Input: part model. Units: mm. Frame: model coordinates. Face numbers are marked on the shaded views. Coordinates: 2 decimals unless noted, no trailing zeros. Loops run counter-clockwise (first coordinate to the right, second up) from the corner with the lowest first, then second, coordinate; pieces in that order, holes last. Notation, with made-up numbers: (53, -21) -> (103, -21) arc R21 ccw to (103, 7) -> close; hole circle Ø4 at (-30, 47). An arc over 180 degrees is marked (long way). Put each result on its own line as item: value. Start each with the question number.
1) Material intervals for L1, parallel to Z at x = 10.25, y = -7.75; L2, parallel to Y at x = 9, z = -19.5; L3, parallel to X at y = 4.75, z = 15, sorted ascending.
2) Cut plane C-C (z = 2.5). Return the cut outline in (x, y), plus the area to 3 significant figures.
3) Pull-direction query (X, two-part tool) for the marked faces 1, 2, 3 and 4; classes: pulls with the +X half, pulls with the -X half, needs draft (parallel to the pull), parting line crosses it, or undercut.
4) Contact query for flat-ended pins moving along their axis: P1, Ø0.5, axis at x = 10.5, y = -2.5, coming from the +Z side; P2, Ø1, axis at x = 4.5, z = -5, coming from the -Y side; P3, Ø2, axis at y = 5, z = 14, coming from the +X side; P4, Ø2.5, axis at x = 11.5, y = -9.5, coming from the +Z side. Output: stop coordinate, or through.
5) Cut plane A-A (z = 15.5). Return the cut outline in (x, y), plus the area to 3 significant figures.
6) Cut plane D-D (x = 6). Return the cut outline in (y, z), plus the area to 4 significant figures.
7) Cut plane B-B (y = 7.25). Return the cut outline in (x, z), plus the area to 3 significant figures.
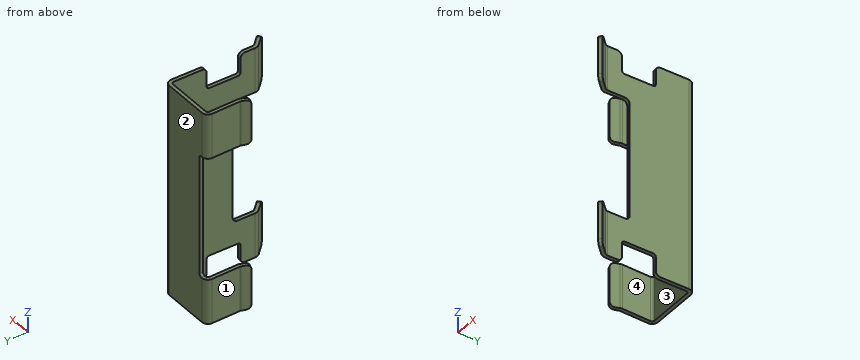
from build123d import *

# Parameters (mm, degrees)
BASE_FLANGE1_DEPTH = 22.5
CUT_EXTRUDE1_START = -9.35
CUT_EXTRUDE1_DEPTH = 9.35
CUT_EXTRUDE2_DEPTH = 28.952537171
FILLET_R1_R        = 1


# Read off the part's stored shape, not the designer's step: Cut-Extrude1
# Sheet-metal steps are written as plain solids
with BuildPart() as part:
    # Sketch1 → Base-Flange1 (new, symmetric)
    with BuildSketch(Plane.XY):
        with BuildLine():
            Line((-0.718242301, 0), (-0.090461069, 1.72481476))
            ThreePointArc((-0.090461069, 1.72481476), (-0.02278837, 1.977372708), (0, 2.237844975))
            Line((0, 2.237844975), (0, 8.1))
            ThreePointArc((0, 8.1), (0.146446609, 8.453553391), (0.5, 8.6))
            Line((0.5, 8.6), (9.985419886, 8.6))
            ThreePointArc((9.985419886, 8.6), (10.344017022, 8.448436644), (10.485213415, 8.085632378))
            Line((10.485213415, 8.085632378), (10.000619414, -8.771503263))
            ThreePointArc((10.000619414, -8.771503263), (10.098258212, -9.348572383), (10.409299492, -9.84434998))
            Line((10.409299492, -9.84434998), (12.522800458, -12.082961625))
            Line((12.522800458, -12.082961625), (13.068150712, -11.568089698))
            Line((13.068150712, -11.568089698), (10.954649746, -9.329478054))
            ThreePointArc((10.954649746, -9.329478054), (10.799129106, -9.081589256), (10.750309707, -8.793054696))
            Line((10.750309707, -8.793054696), (11.234903709, 8.064080946))
            ThreePointArc((11.234903709, 8.064080946), (10.881912725, 8.971091609), (9.985419886, 9.35))
            Line((9.985419886, 9.35), (0.5, 9.35))
            ThreePointArc((0.5, 9.35), (-0.383883476, 8.983883476), (-0.75, 8.1))
            Line((-0.75, 8.1), (-0.75, 2.237844975))
            ThreePointArc((-0.75, 2.237844975), (-0.761394185, 2.107608841), (-0.795230534, 1.981329867))
            Line((-0.795230534, 1.981329867), (-1.423011767, 0.256515107))
            Line((-1.423011767, 0.256515107), (-0.718242301, 0))
        make_face()
    extrude(amount=BASE_FLANGE1_DEPTH, both=True)

    # Cut-Extrude1 outline → Cut-Extrude1 (cut)
    with BuildSketch(Plane(origin=(0, 9.35, 0), x_dir=(-1, 0, 0), z_dir=(0, 1, 0)).offset(CUT_EXTRUDE1_START)):
        with BuildLine():
            ThreePointArc((-0.75, 13), (-1.103553391, 12.853553391), (-1.25, 12.5))
            Line((-1.25, 12.5), (-1.25, -12.5))
            ThreePointArc((-1.25, -12.5), (-1.103553391, -12.853553391), (-0.75, -13))
            Line((-0.75, -13), (3, -13))
            Line((3, -13), (3, 13))
            Line((3, 13), (-0.75, 13))
        make_face()
    extrude(amount=CUT_EXTRUDE1_DEPTH, mode=Mode.SUBTRACT)

    # Sketch5 → Cut-Extrude2 (cut, through all)
    with BuildSketch(Plane(origin=(10.244308957, -0.294494318, 0), x_dir=(0, 0, -1), z_dir=(0.999587057638364, -0.02873524320200468, 0))):
        with BuildLine():
            Line((-22.5, 1.533588636), (-18.5, 1.533588636))
            ThreePointArc((-18.5, 1.533588636), (-18.146446609, 1.387142026), (-18, 1.033588636))
            Line((-18, 1.033588636), (-18, -4.966411364))
            ThreePointArc((-18, -4.966411364), (-18.146446609, -5.319964755), (-18.5, -5.466411364))
            Line((-18.5, -5.466411364), (-22.5, -5.466411364))
            Line((-22.5, -5.466411364), (-22.5, 1.533588636))
        make_face()
        with BuildLine():
            Line((18, 1.033588636), (18, -4.966411364))
            ThreePointArc((18, -4.966411364), (18.146446609, -5.319964755), (18.5, -5.466411364))
            Line((18.5, -5.466411364), (22.5, -5.466411364))
            Line((22.5, -5.466411364), (22.5, 1.533588636))
            Line((22.5, 1.533588636), (18.5, 1.533588636))
            ThreePointArc((18.5, 1.533588636), (18.146446609, 1.387142026), (18, 1.033588636))
        make_face()
        with BuildLine():
            Line((-12, -3.866411364), (12, -3.866411364))
            ThreePointArc((12, -3.866411364), (12.707106781, -4.159304583), (13, -4.866411364))
            Line((13, -4.866411364), (13, -11.718126341))
            Line((13, -11.718126341), (-13, -11.718126341))
            Line((-13, -11.718126341), (-13, -4.866411364))
            ThreePointArc((-13, -4.866411364), (-12.707106781, -4.159304583), (-12, -3.866411364))
        make_face()
    extrude(amount=CUT_EXTRUDE2_DEPTH, mode=Mode.SUBTRACT)

    # R1
    fillet_r1_edges = [part.edges().sort_by_distance(p)[0] for p in [
        (10.663222146, 1.227685317, -22.5),
        (10.462075444, -5.769424086, -22.5),
        (-1.070627034, 0.128257554, -22.5),
        (12.795475585, -11.825525661, 13),
        (12.795475585, -11.825525661, -13),
        (10.663222146, 1.227685317, 22.5),
        (10.462075444, -5.769424086, 22.5),
        (12.795475585, -11.825525661, -22.5),
        (-1.070627034, 0.128257554, 22.5),
        (12.795475585, -11.825525661, 22.5),
        (-1.070627034, 0.128257554, 13),
        (-1.070627034, 0.128257554, -13),
    ]]
    fillet(fillet_r1_edges, radius=FILLET_R1_R)


solid = part.part
Results found:
1. L1: z = -22.5 to -13, 13 to 22.5
1. L2: y = 8.6 to 9.35
1. L3: x = -0.75 to 0, 10.39 to 11.14
2. outline: (1.25, 8.6) -> (9.99, 8.6) arc R0.5 cw to (10.49, 8.09) -> (10.13, -4.16) -> (10.88, -4.18) -> (11.23, 8.06) arc R1.25 ccw to (9.99, 9.35) -> (1.25, 9.35) -> close
2. area: 16.8 mm2
3. face 1: pulls with the -X half
3. face 2: needs draft
3. face 3: undercut
3. face 4: undercut
4. P1: stops at z = 18
4. P2: stops at y = 8.6
4. P3: stops at x = 11.18
4. P4: stops at z = 22.5
5. outline: (-1.42, 0.26) -> (-0.72, 0) -> (-0.09, 1.72) arc R1.5 ccw to (0, 2.24) -> (0, 8.1) arc R0.5 cw to (0.5, 8.6) -> (9.99, 8.6) arc R0.5 cw to (10.49, 8.09) -> (10, -8.77) arc R1.5 ccw to (10.41, -9.84) -> (12.52, -12.08) -> (13.07, -11.57) -> (10.95, -9.33) arc R0.75 cw to (10.75, -8.79) -> (11.23, 8.06) arc R1.25 ccw to (9.99, 9.35) -> (0.5, 9.35) arc R1.25 ccw to (-0.75, 8.1) -> (-0.75, 2.24) arc R0.75 cw to (-0.8, 1.98) -> close
5. area: 30.9 mm2
6. outline: (8.6, -22.5) -> (9.35, -22.5) -> (9.35, 22.5) -> (8.6, 22.5) -> close
6. area: 33.75 mm2
7. outline: (-0.75, -22.5) -> (0, -22.5) -> (0, -13) -> (-0.75, -13) -> close; (-0.75, 13) -> (0, 13) -> (0, 22.5) -> (-0.75, 22.5) -> close; (10.46, -22.5) -> (11.21, -22.5) -> (11.21, 22.5) -> (10.46, 22.5) -> close
7. area: 48.0 mm2
